Autodesk Inventor part; units mm, degrees
ref_plane "YZ Plane" through (0, 0, 0) normal (1, 0, 0) x (0, 1, 0)
ref_plane "XZ Plane" through (0, 0, 0) normal (0, 1, 0) x (-1, 0, 0)
ref_plane "XY Plane" through (0, 0, 0) normal (0, 0, 1) x (1, 0, 0)
sketch "Sketch1" plane through (0, 0, 0) normal (0, 1, 0) x (-1, 0, 0)
  line L0 (9.1659, 4.2179) -> (-600.4341, 4.2179)
  line L1 (-600.4341, 4.2179) -> (-600.4341, -300.5821)
  line L2 (-600.4341, -300.5821) -> (9.1659, -300.5821)
  line L3 (9.1659, -300.5821) -> (9.1659, 4.2179)
  point P0 (0, 0)
  dimension "d0" = 609.6
  dimension "d1" = 304.8
extrude "Extrusion1" add sketch "Sketch1" along normal blind 304.8
sketch "Sketch2" plane through (-9.1659, 0, 4.2179) normal (0, 0, 1) x (1, 0, 0)
  circle A0 centre (101.6, 83.5824) radius 38.1
  circle A1 centre (228.6, 83.5824) radius 38.1
  circle A2 centre (381, 83.5824) radius 38.1
  circle A3 centre (508, 83.5824) radius 38.1
  circle A4 centre (508, 240.9926) radius 38.1
  circle A5 centre (381, 240.9926) radius 38.1
  circle A6 centre (228.6, 240.9926) radius 38.1
  circle A7 centre (101.6, 240.9926) radius 38.1
  line L0 (609.6, 0) -> (609.6, 304.8)
  line L1 (0, 0) -> (0, 304.8)
  point P0 (9.1659, 0)
  dimension "d4" = 76.2
  dimension "d5" = 76.2
  dimension "d6" = 76.2
  dimension "d7" = 76.2
  dimension "d8" = 76.2
  dimension "d9" = 76.2
  dimension "d10" = 76.2
  dimension "d11" = 76.2
  dimension "d12" = 101.6
  dimension "d13" = 127
  dimension "d14" = 101.6
  dimension "d15" = 127
extrude "Extrusion2" add sketch "Sketch2" along normal blind 25.4
properties part number "mapButtonStation"
Can you work these out from the model? Positions are in its coordinate system, mm. A direction names the side the tool comes from. Coordinates: 2 decimals unless noted, no trailing zeros. Loops run counter-clockwise (first coordinate to the right, second up) from the corner with the lowest first, then second, coordinate; pieces in that order, holes last.
Item 1: Suppose I cut it at B-B (x = 235.5). Please give me the cut outline in (y, z).
Answers below:
outline: (0, -300.58) - (304.8, -300.58) - (304.8, 4.22) - (275.54, 4.22) - (275.54, 29.62) - (206.45, 29.62) - (206.45, 4.22) - (118.13, 4.22) - (118.13, 29.62) - (49.04, 29.62) - (49.04, 4.22) - (0, 4.22) - close
Item 2: I'm going to push a flat-ended pin straight in: pin 1 (3 mm diameter, centred on x = 265, y = 47, fed in from +Z). Where does the tip first touch, or does it pass through?
Answers below:
pin 1: stops at z = 4.22
Item 3: Which directions (+Z, -Z, +X, -X, +Y, -Y) give clear straight access to the entire face, cutting with the end or side of a thin tool? Please do faces 4 (the face through (600.434, 150, -146)), 5 (the face through (407.03, 98.17, 16.74)).
Answers below:
face 4: +Z, -Z, +X, +Y, -Y
face 5: +Z
Item 4: Suppose I cut it at D-D (x = 511). Please give me the cut outline in (y, z).
Answers below:
outline: (0, -300.58) - (304.8, -300.58) - (304.8, 4.22) - (277.1, 4.22) - (277.1, 29.62) - (204.89, 29.62) - (204.89, 4.22) - (119.69, 4.22) - (119.69, 29.62) - (47.48, 29.62) - (47.48, 4.22) - (0, 4.22) - close
Item 5: Suppose I cut it at C-C (y = 35). Please give me the cut outline in (x, z), then the cut area to 3 significant figures.
Answers below:
outline: (-9.17, -300.58) - (600.43, -300.58) - (600.43, 4.22) - (-9.17, 4.22) - close
area: 186,000 mm2
Item 6: Suppose I cut it at A-A (y = 98). Please give me the cut outline in (x, z).
Answers below:
outline: (-9.17, -300.58) - (600.43, -300.58) - (600.43, 4.22) - (534.1, 4.22) - (534.1, 29.62) - (463.57, 29.62) - (463.57, 4.22) - (407.1, 4.22) - (407.1, 29.62) - (336.57, 29.62) - (336.57, 4.22) - (254.7, 4.22) - (254.7, 29.62) - (184.17, 29.62) - (184.17, 4.22) - (127.7, 4.22) - (127.7, 29.62) - (57.17, 29.62) - (57.17, 4.22) - (-9.17, 4.22) - close
Item 7: Please list where this line runs through material, in increasing order: L1, parallel to Z at x = 540, y = 252.
Answers below:
L1: z = -300.58 to 4.22
Item 8: If we mould it in two halves opening along Y, with no side actions, what happens to faces 1 (the face through (460.77, 239.32, 16.74)), 2 (the face through (498, 84, 29.618)), 3 (the face through (300, 304.8, -146))? For each: released by +Y, released by -Y, zero draft, split by the parting line, or undercut.
Answers below:
face 1: undercut
face 2: zero draft
face 3: released by +Y
